```python
from build123d import *

# Parameters (mm, degrees)
SKETCH1_R           = 3.25
BOSS_EXTRUDE1_DEPTH = 10
CHAMFER1_SIZE       = 10
CHAMFER2_SIZE       = 5


with BuildPart() as part:
    # Sketch1 → Boss-Extrude1 (new body)
    with BuildSketch(Plane(origin=(0, 0, 0), x_dir=(1, 0, 0), z_dir=(0, 1, 0))):
        Polygon((-7, 23), (-7, -7), (66.5, -7), (66.5, -12), (110.55184454, -12), (110.55184454, 28), (66.5, 28), (66.5, 23), align=None)
        with Locations(Location((0, 0, 0), (0, 0, 270))):
            Circle(SKETCH1_R, mode=Mode.SUBTRACT)
        with Locations(Location((0, 16, 0), (0, 0, 270))):
            Circle(SKETCH1_R, mode=Mode.SUBTRACT)
        with Locations(Location((60, 0, 0), (0, 0, 270))):
            Circle(SKETCH1_R, mode=Mode.SUBTRACT)
        with Locations(Location((60, 16, 0), (0, 0, 270))):
            Circle(SKETCH1_R, mode=Mode.SUBTRACT)
        with BuildLine():
            Line((99.5, 5.8), (94.5, 5.8))
            ThreePointArc((94.5, 5.8), (92.3, 8), (94.5, 10.2))
            Line((94.5, 10.2), (99.5, 10.2))
            ThreePointArc((99.5, 10.2), (101.7, 8), (99.5, 5.8))
        make_face(mode=Mode.SUBTRACT)
        with BuildLine():
            Line((84.5, 11.8), (79.5, 11.8))
            ThreePointArc((79.5, 11.8), (77.3, 14), (79.5, 16.2))
            Line((79.5, 16.2), (84.5, 16.2))
            ThreePointArc((84.5, 16.2), (86.7, 14), (84.5, 11.8))
        make_face(mode=Mode.SUBTRACT)
        with BuildLine():
            Line((84.5, -0.2), (79.5, -0.2))
            ThreePointArc((79.5, -0.2), (77.3, 2), (79.5, 4.2))
            Line((79.5, 4.2), (84.5, 4.2))
            ThreePointArc((84.5, 4.2), (86.7, 2), (84.5, -0.2))
        make_face(mode=Mode.SUBTRACT)
    extrude(amount=BOSS_EXTRUDE1_DEPTH)

    # Chamfer1
    chamfer1_edges = [part.edges().sort_by_distance(p)[0] for p in [
        (110.55184454, 5, -28),
        (110.55184454, 5, 12),
    ]]
    chamfer(chamfer1_edges, length=CHAMFER1_SIZE)

    # Chamfer2
    chamfer2_edges = [part.edges().sort_by_distance(p)[0] for p in [
        (66.5, 5, 12),
        (66.5, 5, -28),
    ]]
    chamfer(chamfer2_edges, length=CHAMFER2_SIZE - 0.0001)  # a hair under: the kernel refuses the full size


solid = part.part
```
For this review, take the finished solid that the model builds, in its own axes (mm). A direction names the side the tool comes from. Round coordinates to 2 decimals unless told otherwise and drop trailing zeros. Write each loop counter-clockwise with the first axis right and the second up, starting at its lowest first coordinate (ties: lowest second). Pieces come first, ordered by that corner, then holes. Notation, with made-up numbers: (89, 51.5) -> (145, 51.5) arc R29 cw to (145, 90.5) -> close; hole circle Ø2 at (-6.5, 3). An arc over 180 degrees is marked (long way). Use one line per item in the form item = value.
1) Take a section at C-C, the plane z = -2. Write out the cut boundary in (x, y), and give its area (3 significant figures).
Found:
outline = (-7, 0) -> (-2.56, 0) -> (-2.56, 10) -> (-7, 10) -> close; (2.56, 0) -> (57.44, 0) -> (57.44, 10) -> (2.56, 10) -> close; (62.56, 0) -> (77.3, 0) -> (77.3, 10) -> (62.56, 10) -> close; (86.7, 0) -> (110.55, 0) -> (110.55, 10) -> (86.7, 10) -> close
area = 979 mm2
2) Take a section at B-B, the plane y = 1.5. Count the separate pieces of the cut face and the enclosed holes in it, and give its area (3 significant figures).
Found:
separate_pieces = 1
enclosed_holes = 7
area = 3,600 mm2
3) Clearance check with flat-ended pins moving along their axes: pin 1 (5 mm diameter, centred on x = 60, z = -16, fed in from -Y); pin 2 (6 mm diameter, centred on x = 15.5, y = 5.5, fed in from +Z); pin 3 (5 mm diameter, centred on x = 34.5, y = 8.5, fed in from -Z); pin 4 (1 mm diameter, centred on y = 4.5, z = 8, fed in from +X). State where each tip first meets the part, or that it passes through.
Found:
pin_1 = through
pin_2 = 7
pin_3 = -23
pin_4 = 105.05
4) To check wall thickness, follow L1, parallel to Z at x = 60.5, y = 9; L2, parallel to X at y = 5.25, z = 3; L3, parallel to X at y = 3.75, z = 0. State the ranges of each line that lie inside material, in increasing order. Write a range as from..to.
Found:
L1 = -23..-19.21, -12.79..-3.21, 3.21..7
L2 = -7..-1.25, 1.25..58.75, 61.25..109.55
L3 = -7..-3.25, 3.25..56.75, 63.25..78.58, 85.42..110.55
5) Mouldability with a two-part tool opening along X and no side actions: class faces 1 (the flat face through (69, 4.9, 9.5)), 2 (the flat face through (105.62, 4.93, -22.93)), 3 (the flat face through (82, 5, -11.8)) as +X half, -X half, draft (parallel to the pull), parting line (faces both ways), or undercut.
Found:
face_1 = -X half
face_2 = +X half
face_3 = undercut
6) Take a section at A-A, the plane x = 0. Write out the cut boundary in (y, z), and give its area (3 significant figures).
Found:
outline = (0, -23) -> (10, -23) -> (10, -19.25) -> (0, -19.25) -> close; (0, -12.75) -> (10, -12.75) -> (10, -3.25) -> (0, -3.25) -> close; (0, 3.25) -> (10, 3.25) -> (10, 7) -> (0, 7) -> close
area = 170 mm2
7) Tool access review of faces 4 (the flat face through (82, 5, 0.2)), 5 (the flat face through (30, 5, -23)), 6 (the flat face through (86, 5, 12)), 7 (the flat face through (29, 5, 7)), 8 (the flat face through (86, 5, -28)): name each direction out of +Z, -Z, +X, -X, +Y, -Y from which nothing blocks a thin tool from reaching the whole face with its end or side.
Found:
face_4 = +Y, -Y
face_5 = -Z, -X, +Y, -Y
face_6 = +Z, +X, -X, +Y, -Y
face_7 = +Z, -X, +Y, -Y
face_8 = -Z, +X, -X, +Y, -Y
8) Take a section at D-D, the plane z = -8. Write out the cut boundary in (x, y).
Found:
outline = (-7, 0) -> (92.3, 0) -> (92.3, 10) -> (-7, 10) -> close; (101.7, 0) -> (110.55, 0) -> (110.55, 10) -> (101.7, 10) -> close
